Model file for the job. Use its own axes, mm. A direction names the side the tool comes from. Give positions to 0.01 mm unless a question says otherwise; leave off trailing zeros. Loops run counter-clockwise (first coordinate to the right, second up) from the corner with the lowest first, then second, coordinate; pieces in that order, holes last. Notation, with made-up numbers: M -31.75,-27 L 26.25,-27 A33 cw 26.25,7 Z; hole C 18,-32 d4. An arc over 180 degrees is marked long. Answer in a Markdown table with one row per item.
```python
from build123d import *

# Parameters (mm, degrees)
F1_DEPTH = 8
F3_DEPTH = 12
F4_R     = 1.5
F5_DEPTH = 20.001


with BuildPart() as f1:
    # F0 (on Front) → F1 (new body)
    with BuildSketch(Plane.XZ):
        with BuildLine():
            Line((6.826992, 11.829606), (8, 11.68729))
            Line((8, 11.68729), (8.825802, 11.587099))
            Line((8.825802, 11.587099), (8.860913, 11.582839))
            Line((8.860913, 11.582839), (31.622957, 7.201101))
            Line((31.622957, 7.201101), (50, 12.781211))
            Line((50, 12.781211), (50, 16))
            Line((50, 16), (8, 16))
            Line((8, 16), (-8, 16))
            Line((-8, 16), (-30, 16))
            Line((-30, 16), (-30, -16))
            Line((-30, -16), (-27.340422, -16))
            Line((-27.340422, -16), (-27.340422, -8.306063))
            Line((-27.340422, -8.306063), (-22.455454, 2.286336))
            Line((-22.455454, 2.286336), (-13.329045, 11.921342))
            ThreePointArc((-13.329045, 11.921342), (-11.915348, 12.964857), (-10.227935, 13.454859))
            ThreePointArc((-10.227935, 13.454859), (-9.96384, 13.475896), (-9.699001, 13.482915))
            Line((-9.699001, 13.482915), (-8, 13.482915))
            Line((-8, 13.482915), (-7.5937, 13.482915))
            Line((-7.5937, 13.482915), (-6.8, 13.482915))
            Line((-6.8, 13.482915), (0, 12.657898))
            Line((0, 12.657898), (6.826992, 11.829606))
        make_face()
        Polygon((0, -16), (0, -14), (-4, -14), (-10.8, -2.733333), (-18.8, -13.4), (-18.8, -16), align=None)
        Polygon((6.128575, -14), (0, -14), (0, -16), (50, -16), (50, -6.804848), (33.646384, -6.804848), align=None)
    extrude(amount=F1_DEPTH)

    # F2 (on face) → F3 (join)
    with BuildSketch(Plane(origin=(0, 0, 0), x_dir=(-1, 0, 0), z_dir=(0, 1, 0))):
        with BuildLine():
            Line((-31.622957, 7.201101), (-50, 12.781211))
            Line((-50, 12.781211), (-50, -6.804848))
            Line((-50, -6.804848), (-33.646384, -6.804848))
            Line((-33.646384, -6.804848), (-6.128575, -14))
            Line((-6.128575, -14), (4, -14))
            Line((4, -14), (10.8, -2.733333))
            Line((10.8, -2.733333), (18.8, -13.4))
            Line((18.8, -13.4), (18.8, -16))
            Line((18.8, -16), (27.340422, -16))
            Line((27.340422, -16), (27.340422, -8.306063))
            Line((27.340422, -8.306063), (22.455454, 2.286336))
            Line((22.455454, 2.286336), (13.329045, 11.921342))
            ThreePointArc((13.329045, 11.921342), (11.674838, 13.07596), (9.699001, 13.482915))
            Line((9.699001, 13.482915), (8, 13.482915))
            Line((8, 13.482915), (6.8, 13.482915))
            Line((6.8, 13.482915), (-8.860913, 11.582839))
            Line((-8.860913, 11.582839), (-31.622957, 7.201101))
        make_face()
        with BuildLine():
            Line((30, -16), (30, 16))
            Line((30, 16), (-50, 16))
            Line((-50, 16), (-50, 12.781211))
            Line((-50, 12.781211), (-31.622957, 7.201101))
            Line((-31.622957, 7.201101), (-8.860913, 11.582839))
            Line((-8.860913, 11.582839), (6.8, 13.482915))
            Line((6.8, 13.482915), (8, 13.482915))
            Line((8, 13.482915), (9.699001, 13.482915))
            ThreePointArc((9.699001, 13.482915), (11.674838, 13.07596), (13.329045, 11.921342))
            Line((13.329045, 11.921342), (22.455454, 2.286336))
            Line((22.455454, 2.286336), (27.340422, -8.306063))
            Line((27.340422, -8.306063), (27.340422, -16))
            Line((27.340422, -16), (30, -16))
        make_face()
        Polygon((-33.646384, -6.804848), (-50, -6.804848), (-50, -16), (18.8, -16), (18.8, -13.4), (10.8, -2.733333), (4, -14), (-6.128575, -14), align=None)
    extrude(amount=F3_DEPTH)

    # F4 (on face) → F5 (cut, through all)
    with BuildSketch(Plane.XZ.offset(8)):
        with Locations((-24, 10)):
            Circle(F4_R)
        with Locations((-10.8, -11)):
            Circle(F4_R)
        with Locations((33.646384, -11)):
            Circle(F4_R)
        with Locations((31.622957, 12)):
            Circle(F4_R)
    extrude(amount=-F5_DEPTH, mode=Mode.SUBTRACT)


solid = f1.part
```
Q1. Drop flat-ended pins along their axis: pin 1 (14.5 mm diameter, centred on x = 11.5, z = -4.5, fed in from -Y); pin 2 (1.5 mm diameter, centred on y = -5, z = -2.5, fed in from +X). Give the stop position or say it passes through.
Reported:
| item | result |
|---|---|
| pin 1 | y = 0 |
| pin 2 | x = -10.49 |
Q2. Probe probe 1 along Z at (x, y) = (-9.5, -2.25); probe 2 along Z at (x, y) = (31.5, 8.75); probe 3 along Z at (x, y) = (-10.8, 4.5). List the from-to ranges inside material, lowest first.
Reported:
| item | result |
|---|---|
| probe 1 | -16 to -11.75, -10.25 to -4.89, 13.48 to 16 |
| probe 2 | -16 to 10.51, 13.49 to 16 |
| probe 3 | -16 to -12.5, -9.5 to 16 |
Q3. Saw through at B-B (x = -24). Give the cut face in (y, z), and give its area (3 significant figures).
Reported:
| item | result |
|---|---|
| outline | M -8,-1.06 L 0,-1.06 L 0,-16 L 12,-16 L 12,8.5 L -8,8.5 Z; M -8,11.5 L 12,11.5 L 12,16 L -8,16 Z |
| area | 461 mm² |
Q4. Saw through at C-C (z = -11). Give the cut face in (x, y), and give its area (3 significant figures).
Reported:
| item | result |
|---|---|
| outline | M -30,-8 L -27.34,-8 L -27.34,0 L -17,0 L -17,-8 L -12.3,-8 L -12.3,12 L -30,12 Z; M -9.3,-8 L -5.81,-8 L -5.81,0 L 17.6,0 L 17.6,-8 L 32.15,-8 L 32.15,12 L -9.3,12 Z; M 35.15,-8 L 50,-8 L 50,12 L 35.15,12 Z |
| area | 1,210 mm² |
Q5. Saw through at D-D (x = 11.5). Give the cut face in (y, z), and give its area (3 significant figures).
Reported:
| item | result |
|---|---|
| outline | M -8,-16 L 12,-16 L 12,16 L -8,16 L -8,11.07 L 0,11.07 L 0,-12.6 L -8,-12.6 Z |
| area | 451 mm² |
Q6. 3-axis set-ups, long thin cutter, end or side, ignore diameter. For faces 4 (the face through (-18.8, -4, -15)), 5 (the face through (42, -4, -6.805)), 6 (the face through (-11.125, 1.86, -12.464)), 7 (the face through (50, 4, 0)), 8 (the face through (-8, -4, 13.483)): which of +Z, -Z, +X, -X, +Y, -Y reach the whole face in a straight line?
Reported:
| item | result |
|---|---|
| face 4 | -Z, -Y |
| face 5 | +X, -Y |
| face 6 | +Y, -Y |
| face 7 | +Z, -Z, +X, +Y, -Y |
| face 8 | -Y |
Q7. Saw through at A-A (y = -6.5). Give the number of separate pieces and of enclosed holes in the cut face, and give its area (3 significant figures).
Reported:
| item | result |
|---|---|
| separate pieces | 2 |
| enclosed holes | 4 |
| area | 1,000 mm² |
Q8. Mould opens along X. For faces 1 (the face through (-14.744, -3.944, -7.992)), 2 (the face through (11, 2, -16)), 3 (the face through (40.68, -3.94, 9.95)) say: released by +X, released by -X, zero draft, split by the parting line, or undercut.
Reported:
| item | result |
|---|---|
| face 1 | undercut |
| face 2 | zero draft |
| face 3 | released by +X |
